Solid Edge part; units mm, degrees
sketch "Sketch1" plane through (0, 0, 0) normal (0, 0, 1) x (1, 0, 0)
  line L0 (4.75, -25) -> (4.75, 25)
  line L1 (4.75, 25) -> (6.25, 25)
  line L2 (6.25, 25) -> (6.25, -25)
  line L3 (6.25, -25) -> (4.75, -25)
revolve "RevolvedProtrusion1" add sketch "Sketch1" angle 360 about axis through (0, 23.3565, 0) along (0, -1, 0)
sketch "Sketch2" plane through (0, 0, 0) normal (0, 0, 1) x (1, 0, 0)
  line L0 (6.25, 31.25) -> (6.25, 25)
  line L1 (4.75, 25) -> (6.25, 25)
  line L2 (4.75, 31.25) -> (4.75, 25)
  line L3 (4.75, 31.25) -> (6.25, 31.25)
  line L4 (6.25, -31.25) -> (6.25, -25)
  line L5 (6.25, -25) -> (4.75, -25)
  line L6 (4.75, -31.25) -> (4.75, -25)
  line L7 (4.75, -31.25) -> (6.25, -31.25)
  circle A0 centre (0, -31.25) radius 6.25
  circle A1 centre (0, -31.25) radius 4.75
  circle A2 centre (0, 31.25) radius 4.75
  circle A3 centre (0, 31.25) radius 6.25
extrude "Protrusion1" add sketch "Sketch2" along normal mid plane 3
Source: CAD feature listing. Evaluate the final solid. Frame: model axes, mm. A direction names the side the tool comes from. Round coordinates to 2 decimals unless told otherwise and drop trailing zeros. Loops run counter-clockwise (first coordinate to the right, second up) from the corner with the lowest first, then second, coordinate; pieces in that order, holes last. Notation, with made-up numbers: M 62.5,63.25 L 84.5,63.25 A35 cw 84.5,95.25 Z; hole C -30,41.5 d8. An arc over 180 degrees is marked long. Use a Markdown table: item, result. Add a question column.
1. Set-up query: faces 1 (the flat face through (3, 27, -1.5)), 2 (the cylindrical face through (-0.62, 35.96, 0.02)), 3 (the cylindrical face through (2.192, 0.35, 4.214)), 4 (the flat face through (3, 27, 1.5)), 5 (the flat face through (4, -28, 1.5)). Return all of +Z, -Z, +X, -X, +Y, -Y with unobstructed straight access to the full face (end or side cutting, diameter ignored); none if empty.
2. Cut plane C-C, the plane z = 4. Output: boundary loops of the cut face in (x, y).
3. Ray query, line 1 along Z through (x, y) = (-0.25, -11) (3 decimals); line 2 along Z through (x, y) = (5.5, -30.5); line 3 along Y through (x, z) = (4.25, 2.5). Return the intervals inside material, ascending. Write a range as [from, to].
4. Cut plane A-A, the plane x = 0. Output: boundary loops of the cut face in (y, z), and give its area (3 significant figures).
5. Contact query for flat-ended pins moving along their axis: pin 1 (6 mm diameter, centred on y = -19, z = 3.5, fed in from +X); pin 2 (0.7 mm diameter, centred on y = -26.5, z = -0.5, fed in from -X); pin 3 (1.5 mm diameter, centred on y = 1.5, z = 5, fed in from -X). Output: stop coordinate, or through.
6. Cut plane D-D, the plane y = -2. Output: boundary loops of the cut face in (x, z), and give its area (3 significant figures).
7. Pull-direction query (X, two-part tool) for faces 6 (the flat face through (6.25, -28, 0)), 7 (the cylindrical face through (-0.62, -35.96, -0.02)), 8 (the flat face through (4, -28, -1.5)); classes: +X half, -X half, draft (parallel to the pull), parting line (faces both ways), or undercut.
8. Cut plane B-B, the plane y = -29.5. Output: boundary loops of the cut face in (x, z).
Solution:
| question | item | result |
|---|---|---|
| 1 | face 1 | -Z, +X, -X, +Y |
| 1 | face 2 | +Z, -Z |
| 1 | face 3 | none |
| 1 | face 4 | +Z, +X, -X, +Y |
| 1 | face 5 | +Z, +X, -X, -Y |
| 2 | outline | M -4.8,-25 L -2.56,-25 L -2.56,25 L -4.8,25 Z; M 2.56,-25 L 4.8,-25 L 4.8,25 L 2.56,25 Z |
| 3 | line 1 | z = [-6.245, -4.743], [4.743, 6.245] |
| 3 | line 2 | z = [-1.5, 1.5] |
| 3 | line 3 | y = [-25, 25] |
| 4 | outline | M -37.5,-1.5 L -36,-1.5 L -36,1.5 L -37.5,1.5 Z; M -26.5,-1.5 L -25,-1.5 L -25,1.5 L -26.5,1.5 Z; M -25,-6.25 L 25,-6.25 L 25,-4.75 L -25,-4.75 Z; M -25,4.75 L 25,4.75 L 25,6.25 L -25,6.25 Z; M 25,-1.5 L 26.5,-1.5 L 26.5,1.5 L 25,1.5 Z; M 36,-1.5 L 37.5,-1.5 L 37.5,1.5 L 36,1.5 Z |
| 4 | area | 168 mm2 |
| 5 | pin 1 | stops at x = 6.23 |
| 5 | pin 2 | stops at x = -4.44 |
| 5 | pin 3 | stops at x = -4.58 |
| 6 | outline | C 0,0 d12.5; hole C 0,0 d9.5 |
| 6 | area | 51.8 mm2 |
| 7 | face 6 | +X half |
| 7 | face 7 | undercut |
| 7 | face 8 | draft |
| 8 | outline | M -6,-1.5 L -4.42,-1.5 L -4.42,1.5 L -6,1.5 Z; M 4.42,-1.5 L 6.25,-1.5 L 6.25,1.5 L 4.42,1.5 Z |
